Geometry: final body of the model. Coordinates: model frame, mm. A direction names the side the tool comes from. Give positions to 0.01 mm unless a question says otherwise; leave off trailing zeros. Write each loop counter-clockwise with the first axis right and the second up, starting at its lowest first coordinate (ties: lowest second). Pieces come first, ordered by that corner, then holes. Notation, with made-up numbers: M 44,54 L 96,54 A26 ccw 96,93 Z; hole C -3,-19 d8. An arc over 180 degrees is marked long. Answer as a JSON object with one key per item and string values.
Autodesk Inventor part; units mm, degrees
ref_plane "YZ Plane" through (0, 0, 0) normal (1, 0, 0) x (0, 1, 0)
ref_plane "XZ Plane" through (0, 0, 0) normal (0, 1, 0) x (-1, 0, 0)
ref_plane "XY Plane" through (0, 0, 0) normal (0, 0, 1) x (1, 0, 0)
sketch "Sketch1" plane through (0, 0, 0) normal (0, 0, 1) x (1, 0, 0)
  line L0 (0, 0) -> (54.61, 0)
  line L1 (54.61, 0) -> (54.61, 29.21)
  line L2 (54.61, 29.21) -> (0, 29.21)
  line L3 (0, 29.21) -> (0, 0)
  dimension "d0" = 54.61
  dimension "d2" = 29.21
extrude "Extrusion1" add sketch "Sketch1" along normal blind 10.16
shell "Shell1" thickness 2.667 removed faces 0
properties part number "LiPo" material "Aluminum 6061"
1) Cut plane B-B on z = 5. Return loops of the section in (x, y), and give its area (3 significant figures).
Geometry check:
{"outline": "M 0,0 L 54.61,0 L 54.61,29.21 L 0,29.21 Z; hole M 2.67,2.67 L 51.94,2.67 L 51.94,26.54 L 2.67,26.54 Z", "area": "419 mm2"}
2) Set-up query: faces 1 (the flat face through (27, 15, 2.667)), 2 (the flat face through (28, 29.21, 5)). Return all of +Z, -Z, +X, -X, +Y, -Y with unobstructed straight access to the full face (end or side cutting, diameter ignored); none if empty.
Geometry check:
{"face 1": "none", "face 2": "+Z, -Z, +X, -X, +Y"}
3) Pull-direction query (X, two-part tool) for faces 3 (the flat face through (27, 0, 5)), 4 (the flat face through (28, 26.543, 5)), 5 (the flat face through (54.61, 14, 5)); classes: pulls with the +X half, pulls with the -X half, needs draft (parallel to the pull), parting line crosses it, or undercut.
Geometry check:
{"face 3": "needs draft", "face 4": "undercut", "face 5": "pulls with the +X half"}
4) Contact query for a flat-ended pin moving along its axis: P1, Ø2.5, axis at x = 37, z = 5.5, coming from the -Y side. Output: stop coordinate, or through.
Geometry check:
{"P1": "stops at y = 0"}
5) Cut plane A-A on y = 19. Return loops of the section in (x, z), and give its area (3 significant figures).
Geometry check:
{"outline": "M 0,0 L 54.61,0 L 54.61,10.16 L 0,10.16 Z; hole M 2.67,2.67 L 51.94,2.67 L 51.94,7.49 L 2.67,7.49 Z", "area": "317 mm2"}
6) Line query: line 1 (Y direction, x = 34.5, z = 6.5); line 2 (Z direction, x = 5.5, y = 22.5); line 3 (X direction, y = 21.5, z = 4). Output: solid intervals per line, ascending. Write a range as from..to.
Geometry check:
{"line 1": "y = 0..2.67, 26.54..29.21", "line 2": "z = 0..2.67, 7.49..10.16", "line 3": "x = 0..2.67, 51.94..54.61"}
